Part model, mm, in its own coordinate system. Coordinates: 2 decimals unless noted, no trailing zeros. Loops run counter-clockwise (first coordinate to the right, second up) from the corner with the lowest first, then second, coordinate; pieces in that order, holes last. Notation, with made-up numbers: M -24.5,17.5 L -0.5,17.5 A18 cw -0.5,24.5 Z; hole C 43.25,62.25 d10. An arc over 180 degrees is marked long. Answer as a JSON object with one key per item and string values. Group by question number.
1. Saw through at C-C on z = 0.4. Write the cut outline in (x, y).
2. Saw through at A-A on y = 5.5. Write the cut outline in (x, z).
3. Drill centre lines: L1, parallel to Y at x = 39.2, z = 0.65; L2, parallel to Y at x = -21.5, z = 0.6; L3, parallel to X at y = 34.5, z = 0.2. Where is each one in solid material? Low to high.
4. Drop a flat-ended pin along its axis: pin 1 Ø3.5 at (x, y) = (39.2, 60) entering from -Z. Give the stop position or say it passes through.
5. Saw through at D-D on y = 60. Write the cut outline in (x, z).
from build123d import *

# Parameters (mm, degrees)
F0_R     = 2.1
F1_DEPTH = 1


with BuildPart() as f1:
    # F0 (on Top) → F1 (new body)
    with BuildSketch(Plane.XY):
        with BuildLine():
            ThreePointArc((65, 39.2), (57.4433549546, 57.4433549546), (39.2, 65))
            Line((39.2, 65), (-39.2, 65))
            ThreePointArc((-39.2, 65), (-57.4433549546, 57.4433549546), (-65, 39.2))
            Line((-65, 39.2), (-65, -39.2))
            ThreePointArc((-65, -39.2), (-57.4433549546, -57.4433549546), (-39.2, -65))
            Line((-39.2, -65), (39.2, -65))
            ThreePointArc((39.2, -65), (57.4433549546, -57.4433549546), (65, -39.2))
            Line((65, -39.2), (65, 39.2))
        make_face()
        with BuildLine():
            ThreePointArc((-57.9, -43.029787234), (-61.4849242405, -44.5147114745), (-60, -40.929787234))
            ThreePointArc((-60, -40.929787234), (-58.5150757595, -41.5448629936), (-57.9, -43.029787234))
        make_face(mode=Mode.SUBTRACT)
        with BuildLine():
            ThreePointArc((62.1, -43.029787234), (58.5150757595, -44.5147114745), (60, -40.929787234))
            ThreePointArc((60, -40.929787234), (61.4849242405, -41.5448629936), (62.1, -43.029787234))
        make_face(mode=Mode.SUBTRACT)
        with BuildLine():
            ThreePointArc((-57.9, 35.370212766), (-58.5150757595, 33.8852885255), (-60, 33.270212766))
            ThreePointArc((-60, 33.270212766), (-61.4849242405, 36.8551370064), (-57.9, 35.370212766))
        make_face(mode=Mode.SUBTRACT)
        with Locations((-39.2, 60)):
            Circle(F0_R, mode=Mode.SUBTRACT)
        with BuildLine():
            ThreePointArc((-55, 39.2), (-50.3722871427, 50.3722871427), (-39.2, 55))
            Line((-39.2, 55), (39.2, 55))
            ThreePointArc((39.2, 55), (50.3722871427, 50.3722871427), (55, 39.2))
            Line((55, 39.2), (55, -39.2))
            ThreePointArc((55, -39.2), (50.3722871427, -50.3722871427), (39.2, -55))
            Line((39.2, -55), (-39.2, -55))
            ThreePointArc((-39.2, -55), (-50.3722871427, -50.3722871427), (-55, -39.2))
            Line((-55, -39.2), (-55, 39.2))
        make_face(mode=Mode.SUBTRACT)
        with BuildLine():
            ThreePointArc((62.1, 35.370212766), (61.4849242405, 33.8852885255), (60, 33.270212766))
            ThreePointArc((60, 33.270212766), (58.5150757595, 36.8551370064), (62.1, 35.370212766))
        make_face(mode=Mode.SUBTRACT)
        with BuildLine():
            ThreePointArc((41.3, 60), (39.2, 57.9), (37.1, 60))
            ThreePointArc((37.1, 60), (39.2, 62.1), (41.3, 60))
        make_face(mode=Mode.SUBTRACT)
        with BuildLine():
            Line((39.2, 55), (-39.2, 55))
            ThreePointArc((-39.2, 55), (-50.3722871427, 50.3722871427), (-55, 39.2))
            Line((-55, 39.2), (-55, -39.2))
            ThreePointArc((-55, -39.2), (-50.3722871427, -50.3722871427), (-39.2, -55))
            Line((-39.2, -55), (39.2, -55))
            ThreePointArc((39.2, -55), (50.3722871427, -50.3722871427), (55, -39.2))
            Line((55, -39.2), (55, 39.2))
            ThreePointArc((55, 39.2), (50.3722871427, 50.3722871427), (39.2, 55))
        make_face()
        with BuildLine():
            ThreePointArc((-53.8, 38.8), (-49.4066017178, 49.4066017178), (-38.8, 53.8))
            Line((-38.8, 53.8), (38.8, 53.8))
            ThreePointArc((38.8, 53.8), (49.4066017178, 49.4066017178), (53.8, 38.8))
            Line((53.8, 38.8), (53.8, -38.8))
            ThreePointArc((53.8, -38.8), (49.4066017178, -49.4066017178), (38.8, -53.8))
            Line((38.8, -53.8), (-38.8, -53.8))
            ThreePointArc((-38.8, -53.8), (-49.4066017178, -49.4066017178), (-53.8, -38.8))
            Line((-53.8, -38.8), (-53.8, 38.8))
        make_face(mode=Mode.SUBTRACT)
    extrude(amount=F1_DEPTH)


solid = f1.part
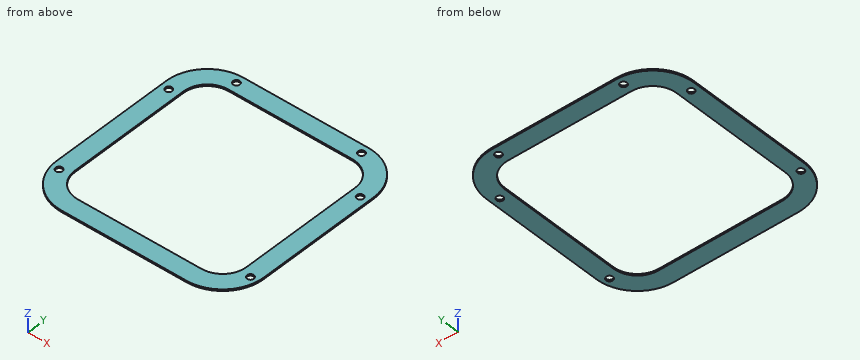
Outcome:
{
 "1": {"outline": "M -65,-39.2 A25.8 ccw -39.2,-65 L 39.2,-65 A25.8 ccw 65,-39.2 L 65,39.2 A25.8 ccw 39.2,65 L -39.2,65 A25.8 ccw -65,39.2 Z; hole C -60,-43.03 d4.2; hole C -60,35.37 d4.2; hole M -53.8,-38.8 A15 ccw -38.8,-53.8 L 38.8,-53.8 A15 ccw 53.8,-38.8 L 53.8,38.8 A15 ccw 38.8,53.8 L -38.8,53.8 A15 ccw -53.8,38.8 Z; hole C -39.2,60 d4.2; hole C 39.2,60 d4.2; hole C 60,-43.03 d4.2; hole C 60,35.37 d4.2"},
 "2": {"outline": "M -65,0 L -53.8,0 L -53.8,1 L -65,1 Z; M 53.8,0 L 65,0 L 65,1 L 53.8,1 Z"},
 "3": {"L1": "y = -65 to -53.79, 53.79 to 57.9, 62.1 to 65", "L2": "y = -65 to -53.8, 53.8 to 65", "L3": "x = -65 to -61.91, -58.09 to -53.8, 53.8 to 58.09, 61.91 to 65"},
 "4": {"pin 1": "passes through"},
 "5": {"outline": "M -54.46,0 L -41.3,0 L -41.3,1 L -54.46,1 Z; M -37.1,0 L 37.1,0 L 37.1,1 L -37.1,1 Z; M 41.3,0 L 54.46,0 L 54.46,1 L 41.3,1 Z"}
}
